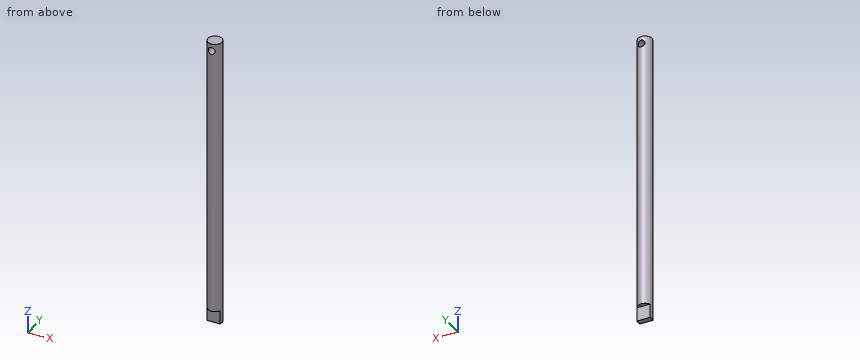
```python
from build123d import *

# Parameters (mm, degrees)
SKETCH1_R           = 3.175
BOSS_EXTRUDE1_DEPTH = 134
CUT_EXTRUDE1_DEPTH  = 6.34
SKETCH5_R           = 1.6
CUT_EXTRUDE2_DEPTH  = 135.187939566


with BuildPart() as part:
    # Sketch1 → Boss-Extrude1 (new body)
    with BuildSketch(Plane.XY):
        Circle(SKETCH1_R)
    extrude(amount=BOSS_EXTRUDE1_DEPTH)

    # Sketch2 → Cut-Extrude1 (cut)
    with BuildSketch(Plane(origin=(0, 0, 0), x_dir=(-1, 0, 0), z_dir=(0, 0, -1))):
        with BuildLine():
            ThreePointArc((2.918582704, 1.25), (0, 3.175), (-2.918582704, 1.25))
            Line((-2.918582704, 1.25), (2.918582704, 1.25))
        make_face()
        with BuildLine():
            Line((2.918582704, -1.25), (-2.918582704, -1.25))
            ThreePointArc((-2.918582704, -1.25), (0, -3.175), (2.918582704, -1.25))
        make_face()
    extrude(amount=-CUT_EXTRUDE1_DEPTH, mode=Mode.SUBTRACT)

    # Sketch5 → Cut-Extrude2 (cut, through all)
    with BuildSketch(Plane(origin=(0, 3.175, 0), x_dir=(1, 0, 0), z_dir=(0, 1, 0))):
        with Locations(Location((0, -130.65, 0), (0, 0, 270))):
            Circle(SKETCH5_R)
    extrude(amount=-CUT_EXTRUDE2_DEPTH, mode=Mode.SUBTRACT)


solid = part.part
```
Build history of the part. All positions in model axes, mm. Round coordinates to 2 decimals unless told otherwise and drop trailing zeros. Write each loop counter-clockwise with the first axis right and the second up, starting at its lowest first coordinate (ties: lowest second). Pieces come first, ordered by that corner, then holes.
1) Drill centre lines: probe 1 along Z at (x, y) = (0, 1); probe 2 along Z at (x, y) = (0, 3); probe 3 along X at (y, z) = (0, 130.65) (3 decimals). Where is each one in solid material? Low to high.
2) Band-saw the part on B-B, the plane z = 100. List the corners of the cut face in (x, y) (3 decimals).
3) Band-saw the part on C-C, the plane z = 130.65. List the corners of the cut face in (x, y) (3 decimals), and give its area (3 significant figures).
4) Band-saw the part on A-A, the plane x = 0. List the corners of the cut face in (y, z) (3 decimals).
5) Pin check, flat tips, straight feed: pin 1 (1 mm diameter, centred on y = 0.5, z = 120.5, fed in from -X) (3 decimals); pin 2 (3 mm diameter, centred on x = 1.5, z = 2, fed in from +Y); pin 3 (1 mm diameter, centred on x = -1, y = 2, fed in from -Z); pin 4 (2 mm diameter, centred on y = -2, z = 99.5, fed in from -X). Stop position of each tip, or through.
Ans:
1. probe 1: z = 0 to 129.05, 132.25 to 134
1. probe 2: z = 6.34 to 129.05, 132.25 to 134
1. probe 3: x = -3.175 to -1.6, 1.6 to 3.175
2. outline: circle Ø6.35 at (0, 0)
3. outline: (-1.6, -2.742) - (-1.6, 2.742) arc R3.175 ccw to start; (1.6, -2.742) arc R3.175 ccw to (1.6, 2.742) - close
3. area: 12.2 mm2
4. outline: (-3.175, 6.34) - (-1.25, 6.34) - (-1.25, 0) - (1.25, 0) - (1.25, 6.34) - (3.175, 6.34) - (3.175, 129.05) - (-3.175, 129.05) - close; (-3.175, 132.25) - (3.175, 132.25) - (3.175, 134) - (-3.175, 134) - close
5. pin 1: stops at x = -3.175
5. pin 2: stops at y = 1.25
5. pin 3: stops at z = 6.34
5. pin 4: stops at x = -3.01
